Read the model definition and answer for the solid it produces. Units are mm, in the model's axes. Give positions to 0.01 mm unless a question says otherwise; leave off trailing zeros.
(1) Straight lines are drawn through the part: probe 1 along Y at (x, z) = (318.5, 13) (3 decimals); probe 2 along Y at (x, z) = (-215, -15) (3 decimals). For each, find the intervals that lie inside material, in ascending order.
(2) Find section A-A, the plane y = 0. State how many separate pieces and enclosed holes the cut face has, then the cut area to 3 significant figures.
(3) Each of these flat-tipped pins is pushed along its axis until it touches: P1, Ø17, axis at x = 317.5, y = 0, coming from the +Z side; P2, Ø12.5, axis at x = -317.5, z = 0, coming from the +Y side. Where does it stop, or does it pass through?
```python
from build123d import *

# Parameters (mm, degrees)
BOSS_EXTRUDE1_DEPTH      = 457.2
BOSS_EXTRUDE1_DEPTH_BACK = 457.2
SKETCH5_R                = 5.334
CUT_EXTRUDE1_DEPTH       = 16.875
SKETCH6_R                = 5.334
CUT_EXTRUDE2_DEPTH       = 16.875
LPATTERN1_COUNT          = 36
LPATTERN1_PITCH          = 25.4


with BuildPart() as part:
    # Sketch4 → Boss-Extrude1 (new body, two sides)
    with BuildSketch(Plane(origin=(0, 0, 0), x_dir=(0, 0, -1), z_dir=(1, 0, 0))) as boss_extrude1_sk:
        with BuildLine():
            Line((-15.875, -13.1318), (11.7602, -13.1318))
            ThreePointArc((11.7602, -13.1318), (12.730067661, -12.730067661), (13.1318, -11.7602))
            Line((13.1318, -11.7602), (13.1318, 15.875))
            Line((13.1318, 15.875), (15.875, 15.875))
            Line((15.875, 15.875), (15.875, -11.7602))
            ThreePointArc((15.875, -11.7602), (14.669802983, -14.669802983), (11.7602, -15.875))
            Line((11.7602, -15.875), (-15.875, -15.875))
            Line((-15.875, -15.875), (-15.875, -13.1318))
        make_face()
    extrude(amount=BOSS_EXTRUDE1_DEPTH)
    extrude(boss_extrude1_sk.sketch, amount=-BOSS_EXTRUDE1_DEPTH_BACK)

    # Sketch5 → Cut-Extrude1 (cut, through all)
    with BuildSketch(Plane.XY):
        with Locations((444.5, 0)):
            Circle(SKETCH5_R)
    cut_extrude1 = extrude(amount=-CUT_EXTRUDE1_DEPTH, mode=Mode.SUBTRACT)

    # Sketch6 → Cut-Extrude2 (cut, through all)
    with BuildSketch(Plane(origin=(0, 0, 0), x_dir=(1, 0, 0), z_dir=(0, 1, 0))):
        with Locations((444.5, 0)):
            Circle(SKETCH6_R)
    cut_extrude2 = extrude(amount=-CUT_EXTRUDE2_DEPTH, mode=Mode.SUBTRACT)

    # LPattern1: Cut-Extrude1, Cut-Extrude2 ×36
    with Locations(*[(-i * LPATTERN1_PITCH, 0, 0) for i in range(1, LPATTERN1_COUNT)]):
        add(cut_extrude1, mode=Mode.SUBTRACT)
        add(cut_extrude2, mode=Mode.SUBTRACT)


solid = part.part
```
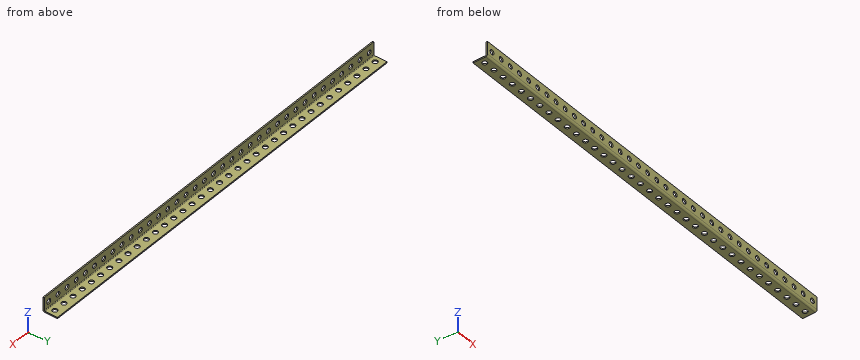
Entries:
1. probe 1: y = -15.875 to -13.132
1. probe 2: y = -14.297 to -5.258, 5.258 to 15.875
2. separate pieces: 37
2. enclosed holes: 0
2. area: 1,450 mm2
3. P1: stops at z = -13.13
3. P2: stops at y = -13.13
